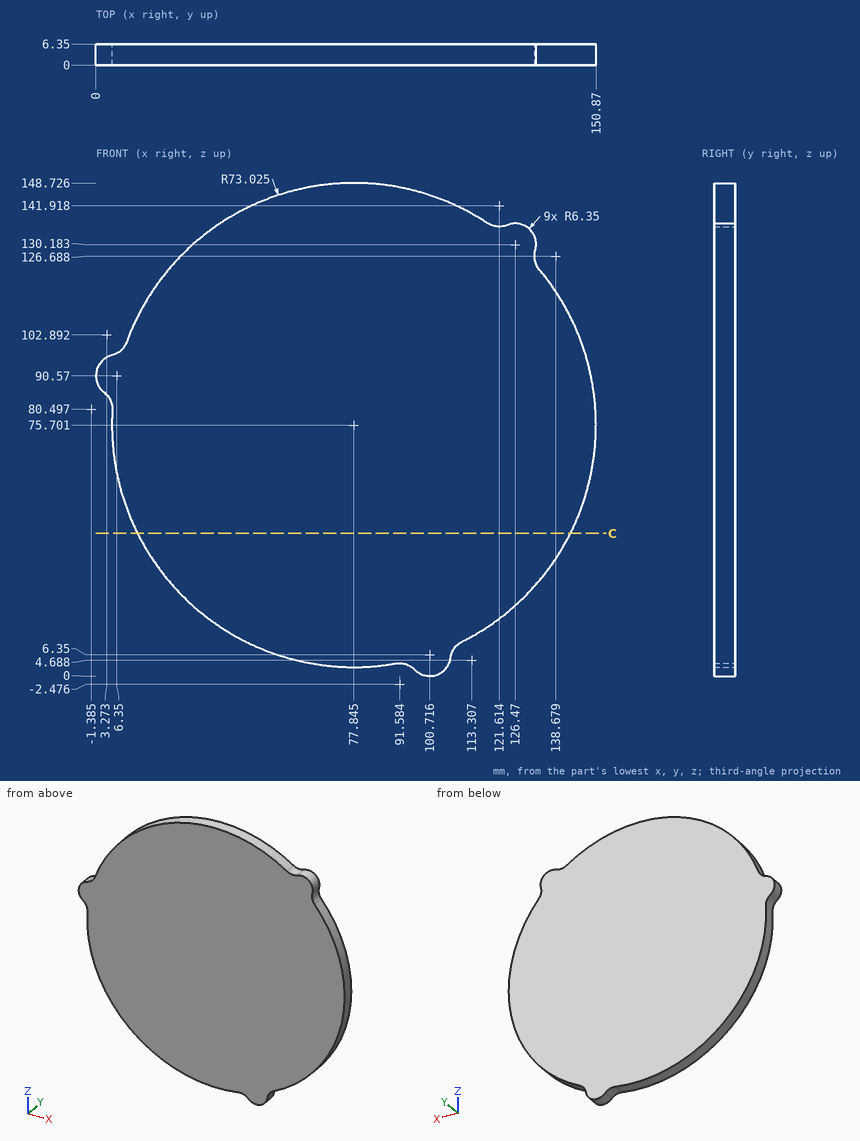
Geometry check sheet. Reference: drawing and pictorial views, mm from the part's lowest x, y, z. Give positions to 0.01 mm unless a question says otherwise; leave off trailing zeros. Order: outer loops, then holes, each group sorted by start corner. A loop starts at its lowest first (then second) coordinate and runs counter-clockwise, first axis right, second up.
1. Gauge pin test, flat end, axial feed: pin 1 Ø2 at (y, z) = (3.5, 111) entering from +X (1 decimal). Record the tip position at first contact, or that the pin passes through.
2. Section check C-C, the plane z = 43. Enter the section's corners in (x, y), and give its area (3 significant figures).
3. Thickness scan on L1, parallel to X at y = 3, z = 74.5; L2, parallel to X at y = 1, z = 132.5; L3, parallel to Z at x = 119, y = 5.25. Record the ranges inside material, lowest first.
Values follow:
1. pin 1: stops at x = 142.3
2. outline: (12.55, 0) - (143.14, 0) - (143.14, 6.35) - (12.55, 6.35) - close
2. area: 829 mm2
3. L1: x = 4.83 to 150.86
3. L2: x = 31.95 to 132.38
3. L3: z = 15.38 to 136.13
